from build123d import *

# Parameters (mm, degrees)
SKETCH_1_W               = 15
SKETCH_1_H               = 15
EXTRUDE_1_DEPTH          = 20
SKETCH_2_W               = 12
SKETCH_2_H               = 12
CUT_EXTRUDE_1_DEPTH      = 17
CUT_EXTRUDE_1_DEPTH_BACK = 0.001


with BuildPart() as part:
    # 草图1 → 凸台-拉伸1 (new body)
    with BuildSketch(Plane.XY):
        Rectangle(SKETCH_1_W, SKETCH_1_H)
    extrude(amount=EXTRUDE_1_DEPTH)

    # 草图2 → 切除-拉伸1 (cut, two sides)
    with BuildSketch(Plane.XY) as cut_extrude_1_sk:
        Rectangle(SKETCH_2_W, SKETCH_2_H)
    extrude(amount=CUT_EXTRUDE_1_DEPTH, mode=Mode.SUBTRACT)
    extrude(cut_extrude_1_sk.sketch, amount=-CUT_EXTRUDE_1_DEPTH_BACK, mode=Mode.SUBTRACT)


solid = part.part
The model under review builds one solid part; all positions refer to its coordinate system, in mm. A direction names the side the tool comes from. Coordinates: 2 decimals unless noted, no trailing zeros. Write each loop counter-clockwise with the first axis right and the second up, starting at its lowest first coordinate (ties: lowest second). Pieces come first, ordered by that corner, then holes. Notation, with made-up numbers: (56, 23) -> (98, 23) arc R23 ccw to (98, 44) -> close; hole circle Ø5 at (39, -2.5). An arc over 180 degrees is marked (long way). Answer in a Markdown table with one row per item.
1. We need section A-A, the plane y = 5.5. State the section outline as (x, z) points.
Answers below:
| item | result |
|---|---|
| outline | (-7.5, 0) -> (-6, 0) -> (-6, 17) -> (6, 17) -> (6, 0) -> (7.5, 0) -> (7.5, 20) -> (-7.5, 20) -> close |
2. We need section B-B, the plane z = 13. State the section outline as (x, y) points, and give its area (3 significant figures).
Answers below:
| item | result |
|---|---|
| outline | (-7.5, -7.5) -> (7.5, -7.5) -> (7.5, 7.5) -> (-7.5, 7.5) -> close; hole (-6, -6) -> (6, -6) -> (6, 6) -> (-6, 6) -> close |
| area | 81.0 mm^2 |
3. For faces 5 (the flat face through (-6, 0, 8)), 6 (the flat face through (-7.5, 0, 10)), list the 3-axis set-ups (+Z, -Z, +X, -X, +Y, -Y) from which the entire face can be reached by the end or side of a thin tool; tool diameter is ignored.
Answers below:
| item | result |
|---|---|
| face 5 | -Z |
| face 6 | +Z, -Z, -X, +Y, -Y |
4. Draft analysis for pull direction X (two halves, no side actions). For faces 1 (the flat face through (7.5, 0, 10)), 2 (the flat face through (6, 0, 8)), 3 (the flat face through (0, 0, 17)), 4 (the flat face through (0, 0, 20)), state which applies: +X half, -X half, draft (parallel to the pull), parting line (faces both ways), or undercut.
Answers below:
| item | result |
|---|---|
| face 1 | +X half |
| face 2 | undercut |
| face 3 | undercut |
| face 4 | draft |
5. Wall thickness on probe 1 along X at (y, z) = (2.25, 12); probe 2 along Z at (x, y) = (0.25, 0.25): over which ranges is each line inside the solid? List them lowest first. Write a range as [from, to].
Answers below:
| item | result |
|---|---|
| probe 1 | x = [-7.5, -6], [6, 7.5] |
| probe 2 | z = [17, 20] |
